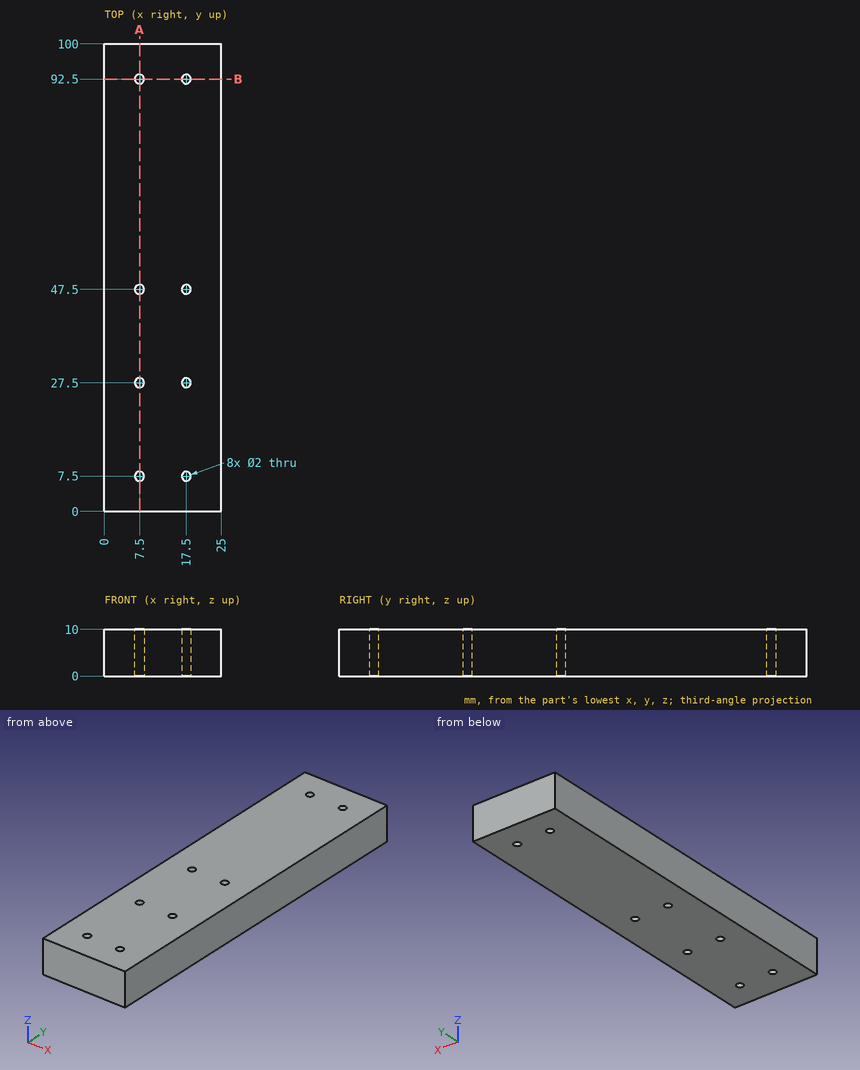
Part print with two shaded views. Sizes in mm from the minimum x, y, z corner. Round coordinates to 2 decimals unless told otherwise and drop trailing zeros. Order: outer loops, then holes, each group sorted by start corner. A loop starts at its lowest first (then second) coordinate and runs counter-clockwise, first axis right, second up. Notation, with made-up numbers: M 22.25,57.5 L 81.25,57.5 A6 ccw 81.25,67.5 Z; hole C -26,-31.5 d1. An arc over 180 degrees is marked long. Put each result on its own line as item: value. Start each with the question number.
1. Slice it at A-A on x = 7.5. List the corners of the cut face in (y, z).
2. Drill centre lines: probe 1 along Y at (x, z) = (17.5, 3.5); probe 2 along X at (y, z) = (92.5, 3.75); probe 3 along Y at (x, z) = (6.75, 7). Where is each one in solid material? Low to high. Write a range as [from, to].
3. Slice it at B-B on y = 92.5. List the corners of the cut face in (x, z).
4. Drop a flat-ended pin along its axis: pin 1 (1.6 mm diameter, centred on x = 7.5, y = 47.5, fed in from +Z). Give the stop position or say it passes through.
Findings:
1. outline: M 0,0 L 6.5,0 L 6.5,10 L 0,10 Z; M 8.5,0 L 26.5,0 L 26.5,10 L 8.5,10 Z; M 28.5,0 L 46.5,0 L 46.5,10 L 28.5,10 Z; M 48.5,0 L 91.5,0 L 91.5,10 L 48.5,10 Z; M 93.5,0 L 100,0 L 100,10 L 93.5,10 Z
2. probe 1: [0, 6.5], [8.5, 26.5], [28.5, 46.5], [48.5, 91.5], [93.5, 100]
2. probe 2: [0, 6.5], [8.5, 16.5], [18.5, 25]
2. probe 3: [0, 6.84], [8.16, 26.84], [28.16, 46.84], [48.16, 91.84], [93.16, 100]
3. outline: M 0,0 L 6.5,0 L 6.5,10 L 0,10 Z; M 8.5,0 L 16.5,0 L 16.5,10 L 8.5,10 Z; M 18.5,0 L 25,0 L 25,10 L 18.5,10 Z
4. pin 1: through
